from build123d import *

# Parameters (mm, degrees)
SKETCH2_W          = 180
SKETCH2_H          = 15
SKETCH3_W          = 32
SKETCH3_H          = 8
CUT_EXTRUDE1_DEPTH = 4.4


with BuildPart() as part:
    # Sketch2 → Revolve1 (revolve)
    with BuildSketch(Plane.XY, mode=Mode.PRIVATE) as revolve1_sk:
        with Locations((90, 7.5)):
            Rectangle(SKETCH2_W, SKETCH2_H)
    revolve(revolve1_sk.sketch.rotate(Axis((0, 0, 0), (-1, 0, 0)), 90), axis=Axis((0, 0, 0), (-1, 0, 0)))

    # Sketch3 → Cut-Extrude1 (cut)
    with BuildSketch(Plane.XY.offset(15)):
        with Locations((143.786391812, 0)):
            Rectangle(SKETCH3_W, SKETCH3_H)
    extrude(amount=-CUT_EXTRUDE1_DEPTH, mode=Mode.SUBTRACT)


solid = part.part
Source: CAD feature listing. Evaluate the final solid. Frame: model axes, mm. A direction names the side the tool comes from. Round coordinates to 2 decimals unless told otherwise and drop trailing zeros. Write each loop counter-clockwise with the first axis right and the second up, starting at its lowest first coordinate (ties: lowest second). Pieces come first, ordered by that corner, then holes. Notation, with made-up numbers: (6, 23.25) - (50, 23.25) arc R35 cw to (50, 60.25) - close; hole circle Ø2 at (61.25, -19). An arc over 180 degrees is marked (long way). Use CSV: the item, a comma, the result in double quotes. Start each with the question number.
(1) Set-up query: faces 1 (the face through (144, -4, 13)), 2 (the face through (180, 0, 0)). Return all of +Z, -Z, +X, -X, +Y, -Y with unobstructed straight access to the full face (end or side cutting, diameter ignored); none if empty.
(2) Cut plane B-B, the plane x = 132.5. Return loops of the section in (y, z).
(3) Mould query, pull axis X, two halves, no side actions, for faces 3 (the face through (127.786, 0, 13)), 4 (the face through (0, 0, 0)), 5 (the face through (91.26, -4.506, -14.307)), 6 (the face through (144, 4, 13)). Classes: pulls with the +X half, pulls with the -X half, needs draft (parallel to the pull), parting line crosses it, or undercut.
(4) First-contact query: pin 1 Ø2.5 at (x, y) = (137.5, -0.5) entering from +Z; pin 2 Ø3 at (x, z) = (146, 12) entering from +Y; pin 3 Ø1 at (x, y) = (28.5, 5) entering from +Z. Flat tips, straight axial feed; report the tip coordinate or a pass-through.
(5) Cut plane C-C, the plane z = -4.25. Return loops of the section in (x, y), and give its area (3 significant figures).
(6) Cut plane A-A, the plane y = 0. Return loops of the section in (x, z).
(7) Material intervals for probe 1 along Z at (x, y) = (41, -0.75); probe 2 along X at (y, z) = (3.5, 13.25); probe 3 along Z at (x, y) = (47, 2), sorted ascending. Write a range as [from, to].
(8) Cut plane D-D, the plane x = 17. Return loops of the section in (y, z).
Geometry says:
1,face 1,"+Z"
1,face 2,"+Z, -Z, +X, +Y, -Y"
2,outline,"(-4, 10.6) - (-4, 14.46) arc R15 ccw (long way) to (4, 14.46) - (4, 10.6) - close"
3,face 3,"undercut"
3,face 4,"pulls with the -X half"
3,face 5,"needs draft"
3,face 6,"undercut"
4,pin 1,"z = 10.6"
4,pin 2,"y = 10.71"
4,pin 3,"z = 14.31"
5,outline,"(0, -14.39) - (180, -14.39) - (180, 14.39) - (0, 14.39) - close"
5,area,"5,180 mm²"
6,outline,"(0, -15) - (180, -15) - (180, 15) - (159.79, 15) - (159.79, 10.6) - (127.79, 10.6) - (127.79, 15) - (0, 15) - close"
7,probe 1,"[-14.98, 14.98]"
7,probe 2,"[0, 127.79], [159.79, 180]"
7,probe 3,"[-14.87, 14.87]"
8,outline,"circle Ø30 at (0, 0)"
